from build123d import *

# Parameters (mm, degrees)
ESQUISSE1_R             = 7.6
BOSS_EXTRU_1_DEPTH      = 8
ESQUISSE2_R             = 11.1
ENL_V_MAT_EXTRU_1_DEPTH = 6.5
ENL_V_MAT_EXTRU_2_REACH = 10
ESQUISSE3_R             = 0.8
ESQUISSE4_R             = 1.5
ENL_V_MAT_EXTRU_3_DEPTH = 15


with BuildPart() as part:
    # Esquisse1 → Boss.-Extru.1 (new body)
    with BuildSketch(Plane.XY):
        with BuildLine():
            Line((-14, 0), (-14, -26))
            Line((-14, -26), (14, -26))
            Line((14, -26), (14, 0))
            ThreePointArc((14, 0), (0, 14), (-14, 0))
        make_face()
        Circle(ESQUISSE1_R, mode=Mode.SUBTRACT)
    extrude(amount=BOSS_EXTRU_1_DEPTH)

    # Esquisse2 → Enlèv. mat.-Extru.1 (cut)
    with BuildSketch(Plane.XY.offset(8)):
        Circle(ESQUISSE2_R)
    extrude(amount=-ENL_V_MAT_EXTRU_1_DEPTH, mode=Mode.SUBTRACT)

    # Esquisse3 → Enlèv. mat.-Extru.2 (cut, up to next)
    with BuildSketch(Plane(origin=(0, 0, 0), x_dir=(-1, 0, 0), z_dir=(0, 0, -1)), mode=Mode.PRIVATE) as enl_v_mat_extru_2_sk1:
        with Locations((0, 9.5)):
            Circle(ESQUISSE3_R)
    enl_v_mat_extru_2_tool1 = extrude(enl_v_mat_extru_2_sk1.sketch, amount=-ENL_V_MAT_EXTRU_2_REACH, mode=Mode.PRIVATE) & part.part
    add(enl_v_mat_extru_2_tool1.solids().sort_by_distance((0, 9.5, 0))[0], mode=Mode.SUBTRACT)
    # Esquisse3 → Enlèv. mat.-Extru.2 (cut, up to next)
    with BuildSketch(Plane(origin=(0, 0, 0), x_dir=(-1, 0, 0), z_dir=(0, 0, -1)), mode=Mode.PRIVATE) as enl_v_mat_extru_2_sk2:
        with Locations((8.227241336, 4.75)):
            Circle(ESQUISSE3_R)
    enl_v_mat_extru_2_tool2 = extrude(enl_v_mat_extru_2_sk2.sketch, amount=-ENL_V_MAT_EXTRU_2_REACH, mode=Mode.PRIVATE) & part.part
    add(enl_v_mat_extru_2_tool2.solids().sort_by_distance((-8.227241, 4.75, 0))[0], mode=Mode.SUBTRACT)
    # Esquisse3 → Enlèv. mat.-Extru.2 (cut, up to next)
    with BuildSketch(Plane(origin=(0, 0, 0), x_dir=(-1, 0, 0), z_dir=(0, 0, -1)), mode=Mode.PRIVATE) as enl_v_mat_extru_2_sk3:
        with Locations((8.227241336, -4.75)):
            Circle(ESQUISSE3_R)
    enl_v_mat_extru_2_tool3 = extrude(enl_v_mat_extru_2_sk3.sketch, amount=-ENL_V_MAT_EXTRU_2_REACH, mode=Mode.PRIVATE) & part.part
    add(enl_v_mat_extru_2_tool3.solids().sort_by_distance((-8.227241, -4.75, 0))[0], mode=Mode.SUBTRACT)
    # Esquisse3 → Enlèv. mat.-Extru.2 (cut, up to next)
    with BuildSketch(Plane(origin=(0, 0, 0), x_dir=(-1, 0, 0), z_dir=(0, 0, -1)), mode=Mode.PRIVATE) as enl_v_mat_extru_2_sk4:
        with Locations((0, -9.5)):
            Circle(ESQUISSE3_R)
    enl_v_mat_extru_2_tool4 = extrude(enl_v_mat_extru_2_sk4.sketch, amount=-ENL_V_MAT_EXTRU_2_REACH, mode=Mode.PRIVATE) & part.part
    add(enl_v_mat_extru_2_tool4.solids().sort_by_distance((0, -9.5, 0))[0], mode=Mode.SUBTRACT)
    # Esquisse3 → Enlèv. mat.-Extru.2 (cut, up to next)
    with BuildSketch(Plane(origin=(0, 0, 0), x_dir=(-1, 0, 0), z_dir=(0, 0, -1)), mode=Mode.PRIVATE) as enl_v_mat_extru_2_sk5:
        with Locations((-8.227241336, -4.75)):
            Circle(ESQUISSE3_R)
    enl_v_mat_extru_2_tool5 = extrude(enl_v_mat_extru_2_sk5.sketch, amount=-ENL_V_MAT_EXTRU_2_REACH, mode=Mode.PRIVATE) & part.part
    add(enl_v_mat_extru_2_tool5.solids().sort_by_distance((8.227241, -4.75, 0))[0], mode=Mode.SUBTRACT)
    # Esquisse3 → Enlèv. mat.-Extru.2 (cut, up to next)
    with BuildSketch(Plane(origin=(0, 0, 0), x_dir=(-1, 0, 0), z_dir=(0, 0, -1)), mode=Mode.PRIVATE) as enl_v_mat_extru_2_sk6:
        with Locations((-8.227241336, 4.75)):
            Circle(ESQUISSE3_R)
    enl_v_mat_extru_2_tool6 = extrude(enl_v_mat_extru_2_sk6.sketch, amount=-ENL_V_MAT_EXTRU_2_REACH, mode=Mode.PRIVATE) & part.part
    add(enl_v_mat_extru_2_tool6.solids().sort_by_distance((8.227241, 4.75, 0))[0], mode=Mode.SUBTRACT)

    # Esquisse4 → Enlèv. mat.-Extru.3 (cut)
    with BuildSketch(Plane.XZ.offset(26)):
        with Locations((-10, 4)):
            Circle(ESQUISSE4_R)
        with Locations((10, 4)):
            Circle(ESQUISSE4_R)
    extrude(amount=-ENL_V_MAT_EXTRU_3_DEPTH, mode=Mode.SUBTRACT)


solid = part.part
Work out the finished part from the listing and answer in its coordinate system (mm). A direction names the side the tool comes from. Coordinates: 2 decimals unless noted, no trailing zeros. Loops run counter-clockwise (first coordinate to the right, second up) from the corner with the lowest first, then second, coordinate; pieces in that order, holes last. Notation, with made-up numbers: (40, 68.5) -> (79, 68.5) arc R28 ccw to (79, 95.5) -> close; hole circle Ø5 at (67, 68.5). An arc over 180 degrees is marked (long way). Answer as CSV lines item,"result".
1) The part is cut by section D-D (x = 3.5). Give the vertices of the cut face in (y, z), and give its area (3 significant figures).
A:
outline,"(-26, 0) -> (-6.75, 0) -> (-6.75, 1.5) -> (-10.53, 1.5) -> (-10.53, 8) -> (-26, 8) -> close; (6.75, 0) -> (13.56, 0) -> (13.56, 8) -> (10.53, 8) -> (10.53, 1.5) -> (6.75, 1.5) -> close"
area,"159 mm²"
2) The part is cut by section A-A (z = 6). Give the vertices of the cut face in (x, y).
A:
outline,"(-14, -26) -> (14, -26) -> (14, 0) arc R14 ccw to (-14, 0) -> close; hole circle Ø22.2 at (0, 0)"
3) Flat-ended cylindrical pins translate along their axes: pin 1 (5 mm diameter, centred on x = -9, y = -5.5, fed in from +Z); pin 2 (1 mm diameter, centred on x = 0, y = -9.5, fed in from -Z); pin 3 (1.5 mm diameter, centred on y = 6, z = 5.5, fed in from +X); pin 4 (2.5 mm diameter, centred on x = 10, z = 4, fed in from -Y). Find the tip coordinate at first contact, or state that the pin passes through.
A:
pin 1,"stops at z = 8"
pin 2,"passes through"
pin 3,"stops at x = 12.98"
pin 4,"stops at y = -11"
4) The part is cut by section B-B (x = 0). Give the vertices of the cut face in (y, z).
A:
outline,"(-26, 0) -> (-10.3, 0) -> (-10.3, 1.5) -> (-11.1, 1.5) -> (-11.1, 8) -> (-26, 8) -> close; (-8.7, 0) -> (-7.6, 0) -> (-7.6, 1.5) -> (-8.7, 1.5) -> close; (7.6, 0) -> (8.7, 0) -> (8.7, 1.5) -> (7.6, 1.5) -> close; (10.3, 0) -> (14, 0) -> (14, 8) -> (11.1, 8) -> (11.1, 1.5) -> (10.3, 1.5) -> close"
5) For a pull along X with two mould halves and no side action, classify faces 4 (the face through (8.5, -18.6, 4.07)), 5 (the face through (0, 14, 4)), 6 (the face through (0, -15, 8)) as released by +X, released by -X, zero draft, split by the parting line, or undercut.
A:
face 4,"undercut"
face 5,"split by the parting line"
face 6,"zero draft"
6) Straight lines are drawn through the part: probe 1 along Y at (x, z) = (0, 0.95); probe 2 along Z at (x, y) = (-10, -14.25); probe 3 along X at (y, z) = (-12, 5). For each, find the intervals that lie inside material, in ascending order.
A:
probe 1,"y = -26 to -10.3, -8.7 to -7.6, 7.6 to 8.7, 10.3 to 14"
probe 2,"z = 0 to 2.5, 5.5 to 8"
probe 3,"x = -14 to -11.12, -8.88 to 8.88, 11.12 to 14"
7) The part is cut by section C-C (y = 4.75). Give the vertices of the cut face in (x, z).
A:
outline,"(-13.17, 0) -> (-9.03, 0) -> (-9.03, 1.5) -> (-10.03, 1.5) -> (-10.03, 8) -> (-13.17, 8) -> close; (-7.43, 0) -> (-5.93, 0) -> (-5.93, 1.5) -> (-7.43, 1.5) -> close; (5.93, 0) -> (7.43, 0) -> (7.43, 1.5) -> (5.93, 1.5) -> close; (9.03, 0) -> (13.17, 0) -> (13.17, 8) -> (10.03, 8) -> (10.03, 1.5) -> (9.03, 1.5) -> close"
8) For faces 1 (the face through (5.97, 9.36, 4.8)), 2 (the face through (0, -26, 4)), 3 (the face through (-10, -11, 4)), determine the directions among +Z, -Z, +X, -X, +Y, -Y from which every point of the face is accessible in a straight line to the end or side of a thin tool.
A:
face 1,"+Z"
face 2,"+Z, -Z, +X, -X, -Y"
face 3,"-Y"
